from build123d import *

# Parameters (mm, degrees)
SKETCH1_R           = 2.15
BOSS_EXTRUDE1_DEPTH = 4.7625
FILLET1_R           = 10
SKETCH2_W           = 4.7625
SKETCH2_H           = 33.783
CUT_EXTRUDE1_DEPTH  = 10


with BuildPart() as part:
    # Sketch1 → Boss-Extrude1 (new body)
    with BuildSketch(Plane(origin=(0, 0, 0), x_dir=(1, 0, 0), z_dir=(0, 1, 0))):
        Polygon((0, 0), (-92, 92), (-92, 110), (-56.601944845, 110), (0, 94.833554589), (0, 58.293), (8, 58.293), (8, -58.293), (0, -58.293), (0, -94.833554589), (-56.601944845, -110), (-92, -110), (-92, -92), align=None)
        with Locations((-85.159917522, 94.147890435)):
            Circle(SKETCH1_R, mode=Mode.SUBTRACT)
        with Locations((-81.358825255, 103.397306502)):
            Circle(SKETCH1_R, mode=Mode.SUBTRACT)
        with Locations((-36.961628134, 85.152063619)):
            Circle(SKETCH1_R, mode=Mode.SUBTRACT)
        with Locations((-40.762720402, 75.902647552)):
            Circle(SKETCH1_R, mode=Mode.SUBTRACT)
        with Locations((-40.762720402, -75.902647552)):
            Circle(SKETCH1_R, mode=Mode.SUBTRACT)
        with Locations((-36.961628134, -85.152063619)):
            Circle(SKETCH1_R, mode=Mode.SUBTRACT)
        with Locations((-81.358825255, -103.397306502)):
            Circle(SKETCH1_R, mode=Mode.SUBTRACT)
        with Locations((-85.159917522, -94.147890435)):
            Circle(SKETCH1_R, mode=Mode.SUBTRACT)
        with BuildLine():
            Line((-79.322036695, 97.830250065), (-76.328676535, 105.114165218))
            ThreePointArc((-76.328676535, 105.114165218), (-76.087243425, 105.511850251), (-75.735570504, 105.816431091))
            ThreePointArc((-75.735570504, 105.816431091), (-75.067221358, 106.038703614), (-74.371100284, 105.931413788))
            Line((-74.371100284, 105.931413788), (-40.148260837, 91.867372399))
            ThreePointArc((-40.148260837, 91.867372399), (-39.577853455, 91.454176231), (-39.258927152, 90.826178087))
            ThreePointArc((-39.258927152, 90.826178087), (-39.223044121, 90.362329254), (-39.331012268, 89.909796149))
            Line((-39.331012268, 89.909796149), (-42.324372428, 82.625880996))
            Line((-42.324372428, 82.625880996), (-36.219757824, 80.1171601))
            Line((-36.219757824, 80.1171601), (-36.694894357, 78.960983092))
            Line((-36.694894357, 78.960983092), (-42.799508961, 81.469703988))
            Line((-42.799508961, 81.469703988), (-45.792869122, 74.185788836))
            ThreePointArc((-45.792869122, 74.185788836), (-46.034302231, 73.788103802), (-46.385975153, 73.483522962))
            ThreePointArc((-46.385975153, 73.483522962), (-47.054324299, 73.261250439), (-47.750445372, 73.368540266))
            Line((-47.750445372, 73.368540266), (-81.973284819, 87.432581654))
            ThreePointArc((-81.973284819, 87.432581654), (-82.543692202, 87.845777823), (-82.862618505, 88.473775966))
            ThreePointArc((-82.862618505, 88.473775966), (-82.898501536, 88.937624799), (-82.790533389, 89.390157905))
            Line((-82.790533389, 89.390157905), (-79.797173228, 96.674073057))
            Line((-79.797173228, 96.674073057), (-85.901787832, 99.182793954))
            Line((-85.901787832, 99.182793954), (-85.426651299, 100.338970962))
            Line((-85.426651299, 100.338970962), (-79.322036695, 97.830250065))
        make_face(mode=Mode.SUBTRACT)
        with BuildLine():
            Line((-47.750445372, -73.368540266), (-81.973284819, -87.432581654))
            ThreePointArc((-81.973284819, -87.432581654), (-82.543692202, -87.845777823), (-82.862618505, -88.473775966))
            ThreePointArc((-82.862618505, -88.473775966), (-82.898501536, -88.937624799), (-82.790533389, -89.390157905))
            Line((-82.790533389, -89.390157905), (-79.797173228, -96.674073057))
            Line((-79.797173228, -96.674073057), (-85.901787832, -99.182793954))
            Line((-85.901787832, -99.182793954), (-85.426651299, -100.338970962))
            Line((-85.426651299, -100.338970962), (-79.322036695, -97.830250065))
            Line((-79.322036695, -97.830250065), (-76.328676535, -105.114165218))
            ThreePointArc((-76.328676535, -105.114165218), (-76.087243425, -105.511850251), (-75.735570504, -105.816431091))
            ThreePointArc((-75.735570504, -105.816431091), (-75.067221358, -106.038703614), (-74.371100284, -105.931413788))
            Line((-74.371100284, -105.931413788), (-40.148260837, -91.867372399))
            ThreePointArc((-40.148260837, -91.867372399), (-39.577853455, -91.454176231), (-39.258927152, -90.826178087))
            ThreePointArc((-39.258927152, -90.826178087), (-39.223044121, -90.362329254), (-39.331012268, -89.909796149))
            Line((-39.331012268, -89.909796149), (-42.324372428, -82.625880996))
            Line((-42.324372428, -82.625880996), (-36.219757824, -80.1171601))
            Line((-36.219757824, -80.1171601), (-36.694894357, -78.960983092))
            Line((-36.694894357, -78.960983092), (-42.799508961, -81.469703988))
            Line((-42.799508961, -81.469703988), (-45.792869122, -74.185788836))
            ThreePointArc((-45.792869122, -74.185788836), (-46.034302231, -73.788103802), (-46.385975153, -73.483522962))
            ThreePointArc((-46.385975153, -73.483522962), (-47.054324299, -73.261250439), (-47.750445372, -73.368540266))
        make_face(mode=Mode.SUBTRACT)
    extrude(amount=BOSS_EXTRUDE1_DEPTH)

    # Fillet1
    fillet1_edges = [part.edges().sort_by_distance(p)[0] for p in [
        (-92, 2.38125, -110),
        (-92, 2.38125, 110),
    ]]
    fillet(fillet1_edges, radius=FILLET1_R)

    # Sketch2 → Cut-Extrude1 (cut)
    with BuildSketch(Plane(origin=(0, 0, 0), x_dir=(1, 0, 0), z_dir=(0, 1, 0))):
        Polygon((-4.829629131, 96.127649814), (-17.19282542, 99.440358276), (-18.425451123, 94.840136528), (-6.062254834, 91.527428067), align=None)
        Polygon((-24.920232031, 101.510910637), (-37.283428319, 104.823619098), (-38.516054022, 100.22339735), (-26.152857733, 96.910688889), align=None)
        Polygon((-26.152857733, -96.910688889), (-38.516054022, -100.22339735), (-37.283428319, -104.823619098), (-24.920232031, -101.510910637), align=None)
        Polygon((-6.062254834, -91.527428067), (-18.425451123, -94.840136528), (-17.19282542, -99.440358276), (-4.829629131, -96.127649814), align=None)
        with Locations((5.61875, 33.4015)):
            Rectangle(SKETCH2_W, SKETCH2_H)
        with Locations((5.61875, -33.4015)):
            Rectangle(SKETCH2_W, SKETCH2_H)
    extrude(amount=CUT_EXTRUDE1_DEPTH, mode=Mode.SUBTRACT)


solid = part.part
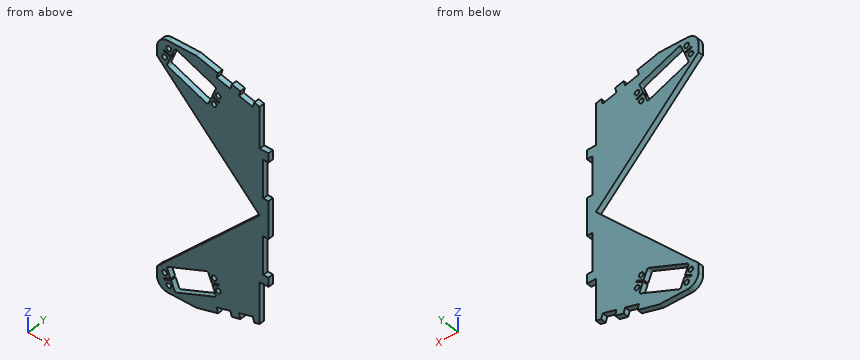
Geometry check sheet. Reference: the model listing, model coordinates, mm. Round coordinates to 2 decimals unless told otherwise and drop trailing zeros. Write each loop counter-clockwise with the first axis right and the second up, starting at its lowest first coordinate (ties: lowest second). Pieces come first, ordered by that corner, then holes.
Item 1: Section check C-C (y = 1.45). Give the number of separate pieces and of enclosed holes in the cut face, plus the area to 3 significant figures.
Determined:
separate pieces: 1
enclosed holes: 10
area: 9,500 mm2
Item 2: Section check D-D (z = -40.5). Record the boundary of the cut face in (x, y), plus the area to 3 significant figures.
Determined:
outline: (-40.5, 0) - (3.24, 0) - (3.24, 4.76) - (-40.5, 4.76) - close
area: 208 mm2
Item 3: Section check B-B (z = 24). Record the boundary of the cut face in (x, y).
Determined:
outline: (-24, 0) - (3.24, 0) - (3.24, 4.76) - (-24, 4.76) - close
Item 4: Go/stop test with flat-tipped pins: pin 1 Ø2.5 at (y, z) = (1.5, -27.5) entering from +X; pin 2 Ø1.4 at (x, y) = (5, 2) entering from -Z; pin 3 Ø1.4 at (x, y) = (6, 3.5) entering from +Z. Record where each tip stops, or that it passes through.
Determined:
pin 1: stops at x = 3.24
pin 2: stops at z = -58.29
pin 3: stops at z = 58.29
Item 5: Material ranges on line 1 along Z through (x, y) = (-65, 1.4); line 2 along Z through (x, y) = (-75.5, 3.1); line 3 along X through (y, z) = (3.45, 74.5), recorded low to high.
Determined:
line 1: z = -110 to -102.08, -80.46 to -65, 65 to 80.46, 102.08 to 110
line 2: z = -110 to -105.94, -84.77 to -75.5, 75.5 to 84.77, 105.94 to 110
line 3: x = -74.5 to -50.5, -45.66 to -42.39, -39.13 to 0
Item 6: Section check A-A (x = -63.5). Record the boundary of the cut face in (y, z), plus the area to 3 significant figures.
Determined:
outline: (0, -110) - (4.76, -110) - (4.76, -101.46) - (0, -101.46) - close; (0, -79.84) - (4.76, -79.84) - (4.76, -63.5) - (0, -63.5) - close; (0, 63.5) - (4.76, 63.5) - (4.76, 79.84) - (0, 79.84) - close; (0, 101.46) - (4.76, 101.46) - (4.76, 110) - (0, 110) - close
area: 237 mm2
